Geometry: final body of the model. Coordinates: model frame, mm. Face numbers are marked on the shaded views. Give positions to 0.01 mm unless a question says otherwise; leave off trailing zeros. Order: outer loops, then holes, each group sorted by start corner. A loop starts at its lowest first (then second) coordinate and runs counter-clockwise, first axis right, second up. Notation, with made-up numbers: (42, 48.5) - (98, 48.5) arc R30 cw to (98, 75.5) - close; hole circle Ø5 at (-17, 68.25). An arc over 180 degrees is marked (long way). Put each result on its own line as item: value. Start each with the question number.
1. Ray query, line 1 along Z through (x, y) = (300, -49); line 2 along Z through (x, y) = (300, -127); line 3 along Z through (x, y) = (-85.5, -35). Return the intervals inside material, ascending. Write a range as from..to.
2. Section D-D on z = -709. Return the cut outline in (x, y).
3. Section C-C on x = 455. Return the cut outline in (y, z), plus the area to 4 significant figures.
4. Section A-A on y = -43.5. Count the separate pieces of the cut face and the enclosed holes in it, plus the area to 3 significant figures.
5. Section B-B on y = -199. Return the cut outline in (x, z), plus the area to 3 significant figures.
6. First-contact query: P1, Ø20.5, axis at x = 0, z = 777.5, coming from the -Y side; P2, Ø2, axis at y = -192.5, z = 364.5, coming from the +X side; P3, Ø5.5, axis at x = 364, z = 722, coming from the -Y side. Flat tips, straight axial feed; report the tip coordinate or a pass-through.
7. Mould query, pull axis X, two halves, no side actions, for the marked faces 1 and 2. Classes: pulls with the +X half, pulls with the -X half, needs draft (parallel to the pull), parting line crosses it, or undercut.
from build123d import *

# Parameters (mm, degrees)
F0_W      = 800
F0_H      = 300
F0_H_2    = 200
F1_DEPTH  = 100
F2_R      = 25
F2_R_2    = 75
F3_DEPTH  = 100
F4_R      = 75
F5_DEPTH  = 150
F6_R      = 82.5
F6_R_2    = 9
F6_R_3    = 25
F7_DEPTH  = 25
F8_R      = 50
F8_R_2    = 25
F9_DEPTH  = 5
F10_R     = 75
F11_DEPTH = 25
F12_R     = 37.5
F13_DEPTH = 100
F14_R     = 92.5
F14_R_2   = 9
F14_R_3   = 37.5
F15_DEPTH = 25
F16_R     = 60
F16_R_2   = 37.5
F17_DEPTH = 5


with BuildPart() as f1:
    # F0 (on Front) → F1 (new body)
    with BuildSketch(Plane.XZ):
        Polygon((400, -965), (550, -965), (550, 965), (-550, 965), (-550, -965), (-400, -965), (-400, -765), (400, -765), align=None)
        with Locations((0, -465)):
            Rectangle(F0_W, F0_H, mode=Mode.SUBTRACT)
        with Locations((0, -65)):
            Rectangle(F0_W, F0_H_2, mode=Mode.SUBTRACT)
    extrude(amount=F1_DEPTH)

    # F2 (on face) → F3 (cut)
    with BuildSketch(Plane.XZ.offset(100)):
        with Locations((-300, 125)):
            Circle(F2_R)
        with Locations((0, 425)):
            Circle(F2_R_2)
        with Locations((-300, 725)):
            Circle(F2_R)
        with Locations((300, 125)):
            Circle(F2_R)
        with Locations((300, 725)):
            Circle(F2_R)
    extrude(amount=-F3_DEPTH, mode=Mode.SUBTRACT)

    # F4 (on face) → F5 (join)
    with BuildSketch(Plane.XZ.offset(100)):
        with Locations((-455, 425)):
            Circle(F4_R)
        with Locations((455, 425)):
            Circle(F4_R)
    extrude(amount=F5_DEPTH)

    # F6 (on face) → F7 (join)
    with BuildSketch(Plane.XZ.offset(100)):
        with Locations((-300, 725)):
            Circle(F6_R)
        with Locations((-300, 662.5)):
            Circle(F6_R_2, mode=Mode.SUBTRACT)
        with Locations((-362.5, 725)):
            Circle(F6_R_2, mode=Mode.SUBTRACT)
        with Locations((-300, 725)):
            Circle(F6_R_3, mode=Mode.SUBTRACT)
        with Locations((-300, 787.5)):
            Circle(F6_R_2, mode=Mode.SUBTRACT)
        with Locations((-237.5, 725)):
            Circle(F6_R_2, mode=Mode.SUBTRACT)
        with Locations((-300, 125)):
            Circle(F6_R)
        with Locations((-300, 62.5)):
            Circle(F6_R_2, mode=Mode.SUBTRACT)
        with Locations((-362.5, 125)):
            Circle(F6_R_2, mode=Mode.SUBTRACT)
        with Locations((-300, 125)):
            Circle(F6_R_3, mode=Mode.SUBTRACT)
        with Locations((-237.5, 125)):
            Circle(F6_R_2, mode=Mode.SUBTRACT)
        with Locations((-300, 187.5)):
            Circle(F6_R_2, mode=Mode.SUBTRACT)
        with Locations((300, 725)):
            Circle(F6_R)
        with Locations((300, 662.5)):
            Circle(F6_R_2, mode=Mode.SUBTRACT)
        with Locations((237.5, 725)):
            Circle(F6_R_2, mode=Mode.SUBTRACT)
        with Locations((300, 725)):
            Circle(F6_R_3, mode=Mode.SUBTRACT)
        with Locations((362.5, 725)):
            Circle(F6_R_2, mode=Mode.SUBTRACT)
        with Locations((300, 787.5)):
            Circle(F6_R_2, mode=Mode.SUBTRACT)
        with Locations((300, 125)):
            Circle(F6_R)
        with Locations((237.5, 125)):
            Circle(F6_R_2, mode=Mode.SUBTRACT)
        with Locations((300, 62.5)):
            Circle(F6_R_2, mode=Mode.SUBTRACT)
        with Locations((300, 125)):
            Circle(F6_R_3, mode=Mode.SUBTRACT)
        with Locations((362.5, 125)):
            Circle(F6_R_2, mode=Mode.SUBTRACT)
        with Locations((300, 187.5)):
            Circle(F6_R_2, mode=Mode.SUBTRACT)
    extrude(amount=F7_DEPTH)

    # F8 (on face) → F9 (join)
    with BuildSketch(Plane.XZ.offset(125)):
        with Locations((-300, 725)):
            Circle(F8_R)
        with Locations((-300, 725)):
            Circle(F8_R_2, mode=Mode.SUBTRACT)
        with Locations((-300, 125)):
            Circle(F8_R)
        with Locations((-300, 125)):
            Circle(F8_R_2, mode=Mode.SUBTRACT)
        with Locations((300, 725)):
            Circle(F8_R)
        with Locations((300, 725)):
            Circle(F8_R_2, mode=Mode.SUBTRACT)
        with Locations((300, 125)):
            Circle(F8_R)
        with Locations((300, 125)):
            Circle(F8_R_2, mode=Mode.SUBTRACT)
    extrude(amount=F9_DEPTH)

    # F10 (on face) → F11 (join)
    with BuildSketch(Plane.XZ.offset(100)):
        with Locations((0, 425)):
            Circle(F10_R)
    extrude(amount=-F11_DEPTH)

    # F12 (on face) → F13 (cut)
    with BuildSketch(Plane.XZ.offset(100)):
        with Locations((0, 850)):
            Circle(F12_R)
    extrude(amount=-F13_DEPTH, mode=Mode.SUBTRACT)

    # F14 (on face) → F15 (join)
    with BuildSketch(Plane.XZ.offset(100)):
        with Locations((0, 850)):
            Circle(F14_R)
        with Locations((-72.5, 850)):
            Circle(F14_R_2, mode=Mode.SUBTRACT)
        with Locations((0, 777.5)):
            Circle(F14_R_2, mode=Mode.SUBTRACT)
        with Locations((0, 850)):
            Circle(F14_R_3, mode=Mode.SUBTRACT)
        with Locations((0, 922.5)):
            Circle(F14_R_2, mode=Mode.SUBTRACT)
        with Locations((72.5, 850)):
            Circle(F14_R_2, mode=Mode.SUBTRACT)
    extrude(amount=F15_DEPTH)

    # F16 (on face) → F17 (join)
    with BuildSketch(Plane.XZ.offset(125)):
        with Locations((0, 850)):
            Circle(F16_R)
        with Locations((0, 850)):
            Circle(F16_R_2, mode=Mode.SUBTRACT)
    extrude(amount=F17_DEPTH)


solid = f1.part
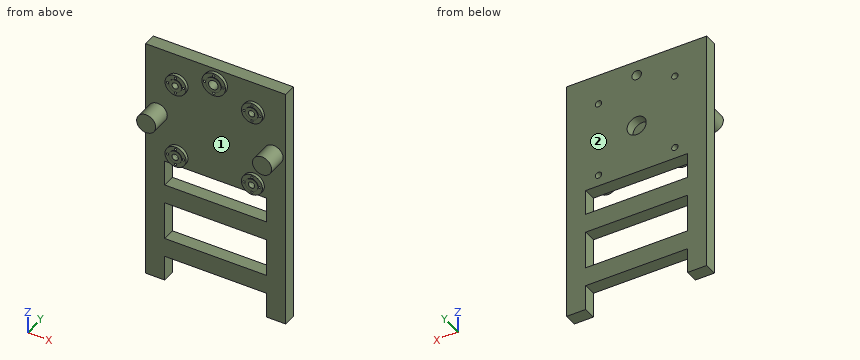
Resolved:
1. line 1: -765..-615, -315..-165, 35..100, 150..700, 750..965
1. line 2: 75..100, 150..175, 675..700, 750..775
1. line 3: -765..-615, -315..-165, 35..965
2. outline: (-550, -100) - (550, -100) - (550, 0) - (-550, 0) - close
3. outline: (-250, 350) - (-100, 350) - (-100, -965) - (0, -965) - (0, 965) - (-100, 965) - (-100, 500) - (-250, 500) - close
3. area: 215,500 mm^2
4. separate pieces: 1
4. enclosed holes: 8
4. area: 1,530,000 mm^2
5. outline: circle Ø150 at (-455, 425); circle Ø150 at (455, 425)
5. area: 35,300 mm^2
6. P1: y = -125
6. P2: x = 500.66
6. P3: y = -100
7. face 1: undercut
7. face 2: needs draft
